Print and shaded views of the part. All mm, measured from the part's lowest x, y and z. A direction names the side the tool comes from. Round coordinates to 2 decimals unless told otherwise and drop trailing zeros. Write each loop counter-clockwise with the first axis right and the second up, starting at its lowest first coordinate (ties: lowest second). Pieces come first, ordered by that corner, then holes. Notation, with made-up numbers: (64, -8) - (76, -8) arc R10 cw to (76, 8) - close; hole circle Ø1 at (36, 77). An arc over 180 degrees is marked (long way). Put each result on its own line as item: value. Start each with the question number.
Item 1: Pin check, flat tips, straight feed: pin 1 Ø0.9 at (x, z) = (2, 1) entering from +Y; pin 2 Ø1.5 at (x, y) = (7.5, 1) entering from -Z; pin 3 Ø0.6 at (y, z) = (2.5, 1) entering from +X; pin 4 Ø0.5 at (x, z) = (2, 1) entering from -Y. Stop position of each tip, or through.
Item 2: Cut at C-C (y = 3.45). Give the cut face in (x, z).
Item 3: Cut at B-B (z = 1.35). Give the cut face in (x, y).
Item 4: Drill centre lines: line 1 (X direction, y = 2.55, z = 0.85); line 2 (Z direction, x = 5.5, y = 2.1); line 3 (Y direction, x = 3, z = 0.3). Where is each one in solid material? Low to high. Write a range as from..to.
Item 5: Cut at D-D (z = 0.75). Give the cut face in (x, y), and give its area (3 significant figures).
Item 6: Mould opens along Y. For the marked faces 4, 5, 6 and 7 say: released by +Y, released by -Y, zero draft, split by the parting line, or undercut.
Item 7: 3-axis set-ups, long thin cutter, end or side, ignore diameter. For the marked faces 1, 2 and 3: which of +Z, -Z, +X, -X, +Y, -Y reach the whole face in a straight line?
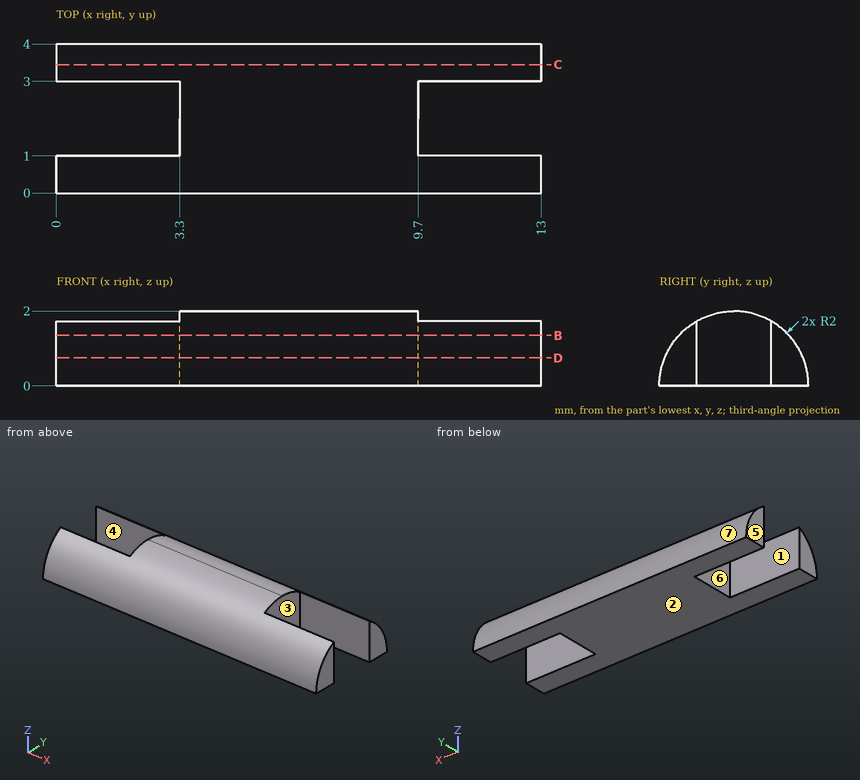
Output values:
1. pin 1: y = 3.92
1. pin 2: z = 0
1. pin 3: x = 9.7
1. pin 4: y = 0.15
2. outline: (0, 0) - (13, 0) - (13, 1.38) - (0, 1.38) - close
3. outline: (0, 0.52) - (13, 0.52) - (13, 1) - (9.7, 1) - (9.7, 3) - (13, 3) - (13, 3.48) - (0, 3.48) - (0, 3) - (3.3, 3) - (3.3, 1) - (0, 1) - close
4. line 1: 3.3..9.7
4. line 2: 0..2
4. line 3: 0.02..1, 3..3.98
5. outline: (0, 0.15) - (13, 0.15) - (13, 1) - (9.7, 1) - (9.7, 3) - (13, 3) - (13, 3.85) - (0, 3.85) - (0, 3) - (3.3, 3) - (3.3, 1) - (0, 1) - close
5. area: 35.0 mm2
6. face 4: undercut
6. face 5: zero draft
6. face 6: undercut
6. face 7: released by +Y
7. face 1: +Z, -Z, -X
7. face 2: -Z, +X, -X, +Y, -Y
7. face 3: +Z, -Z, +X
